Model file for the job. Use its own axes, mm. A direction names the side the tool comes from. Coordinates: 2 decimals unless noted, no trailing zeros. Write each loop counter-clockwise with the first axis right and the second up, starting at its lowest first coordinate (ties: lowest second). Pieces come first, ordered by that corner, then holes. Notation, with made-up numbers: M -6,-9.5 L 20,-9.5 A34 cw 20,26.5 Z; hole C 88,14.5 d5. An arc over 180 degrees is marked long. One line per question, with ' | ' between items. Start each with the question number.
(1) Cut at D-D (x = -58.5). Write the cut outline in (y, z), plus the area to 3 significant figures.
(2) Cut at C-C (y = 9). Write the cut outline in (x, z).
(3) Two-plate mould, pull along X, no slides. Class faces 5 (the face through (36, -36, 25)), 6 (the face through (34.923, 32.226, 4.93)), 7 (the face through (-43, -28, 5)): +X half, -X half, draft (parallel to the pull), parting line (faces both ways), or undercut.
(4) Tool access for faces 1 (the face through (-35, -32, 10)), 2 (the face through (-51, -1, -17)), 3 (the face through (43, -28, 5)), 4 (the face through (57, 20, -13)): list every direction of +Z, -Z, +X, -X, +Y, -Y with a clear straight run to the whole face (end or side of a thin tool).
(5) Cut at B-B (z = 21). Write the cut outline in (x, y).
(6) Cut at A-A (z = -19.5). Write the cut outline in (x, y).
(7) Flat gauge pins, fed straight in: pin 1 Ø5 at (y, z) = (24.5, 4) entering from -X; pin 2 Ø11.5 at (x, z) = (-54, -19) entering from +Y; pin 3 Ø6 at (x, y) = (34, 34) entering from +Z; pin 4 Ø2 at (x, y) = (58.5, -11) entering from +Z. Where does each tip first touch, or does it go through?
(8) Wall check: probe 1 along Y at (x, z) = (-34, 6); probe 2 along Y at (x, z) = (-58.5, -19.5); probe 3 along Y at (x, z) = (34, 22.25). Give the ranges that are in metal, low to high.
from build123d import *

# Parameters (mm, degrees)
SKETCH_1_W          = 86
SKETCH_1_H          = 86
SKETCH_1_R          = 2
EXTRUDE_1_DEPTH     = 10
FILLET_1_R          = 5
SKETCH_2_R          = 9
SKETCH_2_R_2        = 2.5
EXTRUDE_2_DEPTH     = 15
SKETCH_3_R          = 12.5
CUT_EXTRUDE_1_DEPTH = 16
SKETCH_8_W          = 10
SKETCH_8_H          = 42
EXTRUDE_7_DEPTH     = 35
EXTRUDE_7_2_DEPTH   = 35
SKETCH_9_W          = 23
SKETCH_9_H          = 42
EXTRUDE_8_DEPTH     = 10
CUT_EXTRUDE_2_DEPTH = 10
SKETCH_11_W         = 35
SKETCH_11_H         = 42
EXTRUDE_9_DEPTH     = 5
SKETCH_12_W         = 35
SKETCH_12_H         = 42
EXTRUDE_10_DEPTH    = 5
SKETCH_13_R         = 1.75
CUT_EXTRUDE_3_DEPTH = 45


with BuildPart() as part:
    # Sketch 1 → Extrude 1 (new body)
    with BuildSketch(Plane.XY):
        Rectangle(SKETCH_1_W, SKETCH_1_H)
        with Locations((-34, 34)):
            Circle(SKETCH_1_R, mode=Mode.SUBTRACT)
        with Locations((34, 34)):
            Circle(SKETCH_1_R, mode=Mode.SUBTRACT)
        with Locations((34, -34)):
            Circle(SKETCH_1_R, mode=Mode.SUBTRACT)
        with Locations((-34, -34)):
            Circle(SKETCH_1_R, mode=Mode.SUBTRACT)
    extrude(amount=EXTRUDE_1_DEPTH)

    # Fillet 1
    fillet_1_edges = [part.edges().sort_by_distance(p)[0] for p in [
        (-43, 43, 5),
        (43, 43, 5),
        (43, -43, 5),
        (-43, -43, 5),
    ]]
    fillet(fillet_1_edges, radius=FILLET_1_R)

    # Sketch 2 → Extrude 2 (add)
    with BuildSketch(Plane.XY.offset(10)):
        with Locations((-34, 34)):
            Circle(SKETCH_2_R)
        with Locations((-34, 34)):
            Circle(SKETCH_2_R_2, mode=Mode.SUBTRACT)
        with Locations((34, 34)):
            Circle(SKETCH_2_R)
        with Locations((34, 34)):
            Circle(SKETCH_2_R_2, mode=Mode.SUBTRACT)
        with Locations((34, -34)):
            Circle(SKETCH_2_R)
        with Locations((34, -34)):
            Circle(SKETCH_2_R_2, mode=Mode.SUBTRACT)
        with Locations((-34, -34)):
            Circle(SKETCH_2_R)
        with Locations((-34, -34)):
            Circle(SKETCH_2_R_2, mode=Mode.SUBTRACT)
    extrude(amount=EXTRUDE_2_DEPTH)

    # Sketch 3 → Cut-Extrude 1 (cut)
    with BuildSketch(Plane.XY.offset(10)):
        Circle(SKETCH_3_R)
    extrude(amount=-CUT_EXTRUDE_1_DEPTH, mode=Mode.SUBTRACT)



with BuildPart() as body_2:
    # Sketch 8 → Extrude 7 (new body)
    with BuildSketch(Plane(origin=(0, 0, 0), x_dir=(-1, 0, 0), z_dir=(0, 0, -1))):
        with Locations((-61, -1)):
            Rectangle(SKETCH_8_W, SKETCH_8_H)
    extrude(amount=EXTRUDE_7_DEPTH)


with BuildPart() as body_3:
    # Sketch 8 → Extrude 7 2 (new body)
    with BuildSketch(Plane(origin=(0, 0, 0), x_dir=(-1, 0, 0), z_dir=(0, 0, -1))):
        with Locations((61, -1)):
            Rectangle(SKETCH_8_W, SKETCH_8_H)
    extrude(amount=EXTRUDE_7_2_DEPTH)


with BuildPart() as part_1:
    add(part.part)

    add(body_2.part)  # Extrude 8 merges body 2

    add(body_3.part)  # Extrude 8 merges body 3
    # Sketch 9 → Extrude 8 (add)
    with BuildSketch(Plane.XY):
        with Locations((-54.5, -1)):
            Rectangle(SKETCH_9_W, SKETCH_9_H)
        with Locations((54.5, -1)):
            Rectangle(SKETCH_9_W, SKETCH_9_H)
    extrude(amount=EXTRUDE_8_DEPTH)

    # Sketch 10 → Cut-Extrude 2 (cut)
    with BuildSketch(Plane.XY.offset(10)):
        with BuildLine():
            Line((34, 43), (43, 43))
            Line((43, 43), (43, 34))
            ThreePointArc((43, 34), (40.363961031, 40.363961031), (34, 43))
        make_face()
        with BuildLine():
            Line((-43, 43), (-34, 43))
            ThreePointArc((-34, 43), (-40.363961031, 40.363961031), (-43, 34))
            Line((-43, 34), (-43, 43))
        make_face()
        with BuildLine():
            Line((-43, -43), (-34, -43))
            ThreePointArc((-34, -43), (-40.363961031, -40.363961031), (-43, -34))
            Line((-43, -34), (-43, -43))
        make_face()
        with BuildLine():
            Line((34, -43), (43, -43))
            Line((43, -43), (43, -34))
            ThreePointArc((43, -34), (40.363961031, -40.363961031), (34, -43))
        make_face()
    extrude(amount=-CUT_EXTRUDE_2_DEPTH, mode=Mode.SUBTRACT)

    # Sketch 11 → Extrude 9 (add)
    with BuildSketch(Plane.ZY.offset(-56)):
        with Locations((-17.5, -1)):
            Rectangle(SKETCH_11_W, SKETCH_11_H)
    extrude(amount=EXTRUDE_9_DEPTH)

    # Sketch 12 → Extrude 10 (add)
    with BuildSketch(Plane(origin=(-56, 0, 0), x_dir=(0, 0, -1), z_dir=(1, 0, 0))):
        with Locations((17.5, -1)):
            Rectangle(SKETCH_12_W, SKETCH_12_H)
    extrude(amount=EXTRUDE_10_DEPTH)

    # Sketch 13 → Cut-Extrude 3 (cut)
    with BuildSketch(Plane(origin=(0, 0, -35), x_dir=(-1, 0, 0), z_dir=(0, 0, -1))):
        with Locations((58.5, 9)):
            Circle(SKETCH_13_R)
        with Locations((58.5, -1)):
            Circle(SKETCH_13_R)
        with Locations((58.5, -11)):
            Circle(SKETCH_13_R)
        with Locations((-58.5, -11)):
            Circle(SKETCH_13_R)
        with Locations((-58.5, -1)):
            Circle(SKETCH_13_R)
        with Locations((-58.5, 9)):
            Circle(SKETCH_13_R)
    extrude(amount=-CUT_EXTRUDE_3_DEPTH, mode=Mode.SUBTRACT)


solid = part_1.part
Filled in:
1) outline: M -22,-35 L -12.75,-35 L -12.75,10 L -22,10 Z; M -9.25,-35 L -2.75,-35 L -2.75,10 L -9.25,10 Z; M 0.75,-35 L 7.25,-35 L 7.25,10 L 0.75,10 Z; M 10.75,-35 L 20,-35 L 20,10 L 10.75,10 Z | area: 1,420 mm²
2) outline: M -66,-35 L -60.25,-35 L -60.25,10 L -66,10 Z; M -56.75,-35 L -51,-35 L -51,0 L -8.67,0 L -8.67,10 L -56.75,10 Z; M 8.67,0 L 51,0 L 51,-35 L 56.75,-35 L 56.75,10 L 8.67,10 Z; M 60.25,-35 L 66,-35 L 66,10 L 60.25,10 Z
3) face 5: draft | face 6: undercut | face 7: -X half
4) face 1: +Z | face 2: -Z, +Y, -Y | face 3: +Z, -Z, +X, -Y | face 4: +Z, -Z, +X, +Y
5) outline: C -34,-34 d18; C -34,34 d18; C 34,-34 d18; C 34,34 d18; hole C -34,-34 d5; hole C -34,34 d5; hole C 34,-34 d5; hole C 34,34 d5
6) outline: M -66,-22 L -51,-22 L -51,20 L -66,20 Z; M 51,-22 L 66,-22 L 66,20 L 51,20 Z; hole C -58.5,-11 d3.5; hole C -58.5,-1 d3.5; hole C -58.5,9 d3.5; hole C 58.5,-11 d3.5; hole C 58.5,-1 d3.5; hole C 58.5,9 d3.5
7) pin 1: x = -43 | pin 2: y = 20 | pin 3: z = 25 | pin 4: through
8) probe 1: -43 to -36, -32 to 32, 36 to 43 | probe 2: -22 to -12.75, -9.25 to -2.75, 0.75 to 7.25, 10.75 to 20 | probe 3: -43 to -36.5, -31.5 to -25, 25 to 31.5, 36.5 to 43
